from build123d import *

# Parameters (mm, degrees)
F0_W     = 67
F0_H     = 89
F0_W_2   = 3.5
F0_H_2   = 3.5
F0_W_3   = 57
F0_H_3   = 79
F1_DEPTH = 5
F2_R     = 4


with BuildPart() as f1:
    # F0 (on Top) → F1 (new body)
    with BuildSketch(Plane.XY):
        Rectangle(F0_W, F0_H)
        with Locations((-31, -22)):
            Rectangle(F0_W_2, F0_H_2, mode=Mode.SUBTRACT)
        with Locations((31, -22)):
            Rectangle(F0_W_2, F0_H_2, mode=Mode.SUBTRACT)
        Rectangle(F0_W_3, F0_H_3, mode=Mode.SUBTRACT)
        with Locations((-31, 32)):
            Rectangle(F0_W_2, F0_H_2, mode=Mode.SUBTRACT)
        with Locations((31, 32)):
            Rectangle(F0_W_2, F0_H_2, mode=Mode.SUBTRACT)
        with BuildLine():
            Line((-33.5, 44.5), (33.5, 44.5))
            ThreePointArc((33.5, 44.5), (0, 48.5), (-33.5, 44.5))
        make_face()
    extrude(amount=F1_DEPTH)

    # F2
    f2_edges = [f1.edges().sort_by_distance(p)[0] for p in [
        (-33.5, -44.5, 2.5),
        (33.5, -44.5, 2.5),
        (-33.5, 44.5, 2.5),
        (33.5, 44.5, 2.5),
        (-28.5, 39.5, 2.5),
        (28.5, 39.5, 2.5),
        (28.5, -39.5, 2.5),
        (-28.5, -39.5, 2.5),
    ]]
    fillet(f2_edges, radius=F2_R)


solid = f1.part
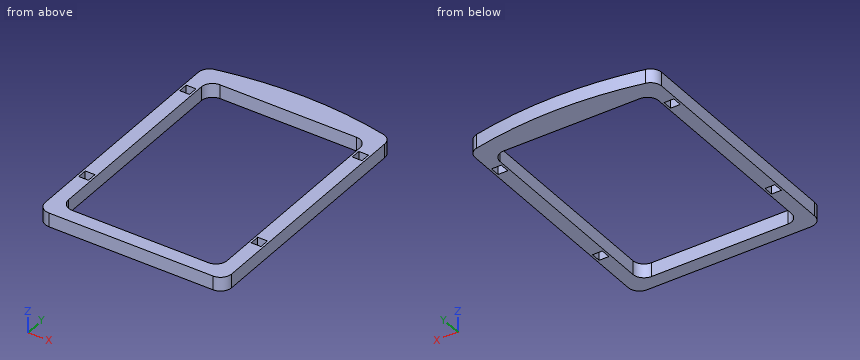
Can you work these out from the model? Positions are in its coordinate system, mm. Give positions to 0.01 mm unless a question says otherwise; leave off trailing zeros. Order: outer loops, then holes, each group sorted by start corner. A loop starts at its lowest first (then second) coordinate and runs counter-clockwise, first axis right, second up. Notation, with made-up numbers: M 7,-40 L 34,-40 A18 ccw 34,-32 Z; hole C 47.25,20 d4. An arc over 180 degrees is marked long. Use one line per item in the form item = value.
Item 1: If we section it at A-A, the plane y = -4: Write out the boundary of the cut face in (x, z), and give its area (3 significant figures).
Values follow:
outline = M -33.5,0 L -28.5,0 L -28.5,5 L -33.5,5 Z; M 28.5,0 L 33.5,0 L 33.5,5 L 28.5,5 Z
area = 50.0 mm^2
Item 2: If we section it at B-B, the plane z = 3.2: Count the separate pieces of the cut face and the enclosed holes in it, and give its area (3 significant figures).
Values follow:
separate_pieces = 1
enclosed_holes = 5
area = 1,590 mm^2
Item 3: Will these pins go through, and if not, where does the flat tip stop? pin 1 Ø1 at (x, z) = (30.5, 2) entering from -Y; pin 2 Ø1.8 at (x, z) = (30.5, 3.5) entering from +Y; pin 3 Ø1.8 at (x, z) = (-31.5, 2.5) entering from -Y.
Values follow:
pin_1 = -44.47
pin_2 = 45.39
pin_3 = -44.35
Item 4: If I drill on line 1 along X through (y, z) = (-34, 3.25); line 2 along Y through (x, z) = (30.5, 1.45); line 3 along Y through (x, z) = (26, 1.2), over which ranges is the centre line in solid material (lowest first)? Write a range as [from, to].
Values follow:
line_1 = [-33.5, -28.5], [28.5, 33.5]
line_2 = [-44.37, -23.75], [-20.25, 30.25], [33.75, 45.19]
line_3 = [-44.5, -39.21], [39.21, 46.1]
Item 5: If we section it at C-C, the plane x = 14: Write out the boundary of the cut face in (y, z).
Values follow:
outline = M -44.5,0 L -39.5,0 L -39.5,5 L -44.5,5 Z; M 39.5,0 L 47.81,0 L 47.81,5 L 39.5,5 Z
